Here's how the part is built. I have some questions about the finished solid (model axes, mm). Face numbers are marked on the shaded views. A direction names the side the tool comes from. Give positions to 0.01 mm unless a question says otherwise; leave off trailing zeros. Write each loop counter-clockwise with the first axis right and the second up, starting at its lowest first coordinate (ties: lowest second). Pieces come first, ordered by that corner, then holes. Notation, with made-up numbers: (-12.75, 10.25) - (-4.75, 10.25) arc R11 ccw to (-4.75, 19.25) - close; hole circle Ø8 at (54, 16). An arc over 180 degrees is marked (long way). Use a Markdown table: item, result.
```python
from build123d import *

# Parameters (mm, degrees)
SKETCH_1_R      = 1.49999994
SKETCH_1_R_2    = 9.999999603
SKETCH_1_R_3    = 2.499999901
EXTRUDE_1_DEPTH = 1.5
SKETCH_2_W      = 1.5
SKETCH_2_H      = 360
EXTRUDE_2_DEPTH = 25


with BuildPart() as part:
    # 草图1 → 凸台-拉伸1 (new body)
    with BuildSketch(Plane.XY):
        with BuildLine():
            Line((124.999995033, 180), (124.999995033, -180))
            Line((124.999995033, -180), (123.499999503, -180))
            Line((123.499999503, -180), (109.999999801, -180))
            ThreePointArc((109.999999801, -180), (106.464466036, -178.535533964), (105, -175.000000199))
            Line((105, -175.000000199), (105, -112.999998311))
            ThreePointArc((105, -112.999998311), (103.535533964, -109.464464546), (100.000000199, -107.99999851))
            Line((100.000000199, -107.99999851), (-250.16001102, -107.99999851))
            ThreePointArc((-250.16001102, -107.99999851), (-253.695544785, -109.464464546), (-255.160010821, -112.999998311))
            Line((-255.160010821, -112.999998311), (-255.160010821, -167.500000497))
            Line((-255.160010821, -167.500000497), (-255.160010821, -175.000000199))
            ThreePointArc((-255.160010821, -175.000000199), (-256.624476857, -178.535533964), (-260.160010622, -180))
            Line((-260.160010622, -180), (-273.660010324, -180))
            Line((-273.660010324, -180), (-275.160005854, -180))
            Line((-275.160005854, -180), (-275.160005854, 180))
            Line((-275.160005854, 180), (-273.660010324, 180))
            Line((-273.660010324, 180), (-260.160010622, 180))
            ThreePointArc((-260.160010622, 180), (-256.624476857, 178.535533964), (-255.160010821, 175.000000199))
            Line((-255.160010821, 175.000000199), (-255.160010821, 112.999998311))
            ThreePointArc((-255.160010821, 112.999998311), (-253.695544785, 109.464464546), (-250.16001102, 107.99999851))
            Line((-250.16001102, 107.99999851), (100.000000199, 107.99999851))
            ThreePointArc((100.000000199, 107.99999851), (103.535533964, 109.464464546), (105, 112.999998311))
            Line((105, 112.999998311), (105, 175.000000199))
            ThreePointArc((105, 175.000000199), (106.464466036, 178.535533964), (109.999999801, 180))
            Line((109.999999801, 180), (123.499999503, 180))
            Line((123.499999503, 180), (124.999995033, 180))
        make_face()
        with Locations((-201.080000404, 97.999998907)):
            Circle(SKETCH_1_R, mode=Mode.SUBTRACT)
        with Locations((-170.080001635, 97.999998907)):
            Circle(SKETCH_1_R, mode=Mode.SUBTRACT)
        Circle(SKETCH_1_R_2, mode=Mode.SUBTRACT)
        with Locations((114.99999543, 31.999998728)):
            Circle(SKETCH_1_R, mode=Mode.SUBTRACT)
        with Locations((82.999996702, 31.999998728)):
            Circle(SKETCH_1_R, mode=Mode.SUBTRACT)
        with Locations((19.919990815, 97.999998907)):
            Circle(SKETCH_1_R, mode=Mode.SUBTRACT)
        with Locations((50.919989583, 97.999998907)):
            Circle(SKETCH_1_R, mode=Mode.SUBTRACT)
        with Locations((19.919990815, 67.000000139)):
            Circle(SKETCH_1_R, mode=Mode.SUBTRACT)
        with Locations((50.919989583, 67.000000139)):
            Circle(SKETCH_1_R, mode=Mode.SUBTRACT)
        with Locations((-201.080000404, -97.999998907)):
            Circle(SKETCH_1_R, mode=Mode.SUBTRACT)
        with Locations((-170.080001635, -97.999998907)):
            Circle(SKETCH_1_R, mode=Mode.SUBTRACT)
        with Locations((19.919990815, -97.999998907)):
            Circle(SKETCH_1_R, mode=Mode.SUBTRACT)
        with Locations((50.919989583, -97.999998907)):
            Circle(SKETCH_1_R, mode=Mode.SUBTRACT)
        with Locations((114.99999543, -31.999998728)):
            Circle(SKETCH_1_R, mode=Mode.SUBTRACT)
        with Locations((82.999996702, -31.999998728)):
            Circle(SKETCH_1_R, mode=Mode.SUBTRACT)
        with Locations((-107.080004139, 97.999998907)):
            Circle(SKETCH_1_R, mode=Mode.SUBTRACT)
        with Locations((-107.080004139, 66.000000179)):
            Circle(SKETCH_1_R, mode=Mode.SUBTRACT)
        with Locations((-43.080006682, 97.999998907)):
            Circle(SKETCH_1_R, mode=Mode.SUBTRACT)
        with Locations((-43.080006682, 66.000000179)):
            Circle(SKETCH_1_R, mode=Mode.SUBTRACT)
        with Locations((-107.080004139, -97.999998907)):
            Circle(SKETCH_1_R, mode=Mode.SUBTRACT)
        with Locations((-107.080004139, -66.000000179)):
            Circle(SKETCH_1_R, mode=Mode.SUBTRACT)
        with Locations((-43.080006682, -97.999998907)):
            Circle(SKETCH_1_R, mode=Mode.SUBTRACT)
        with Locations((-43.080006682, -66.000000179)):
            Circle(SKETCH_1_R, mode=Mode.SUBTRACT)
        with Locations((-201.080000404, 67.000000139)):
            Circle(SKETCH_1_R, mode=Mode.SUBTRACT)
        with Locations((-170.080001635, 67.000000139)):
            Circle(SKETCH_1_R, mode=Mode.SUBTRACT)
        with Locations((-201.080000404, -67.000000139)):
            Circle(SKETCH_1_R, mode=Mode.SUBTRACT)
        with Locations((-170.080001635, -67.000000139)):
            Circle(SKETCH_1_R, mode=Mode.SUBTRACT)
        with Locations((19.919990815, -67.000000139)):
            Circle(SKETCH_1_R, mode=Mode.SUBTRACT)
        with Locations((50.919989583, -67.000000139)):
            Circle(SKETCH_1_R, mode=Mode.SUBTRACT)
        with Locations((-196.080000602, 97.999998907)):
            Circle(SKETCH_1_R, mode=Mode.SUBTRACT)
        with Locations((-196.080000602, 84.999999424)):
            Circle(SKETCH_1_R, mode=Mode.SUBTRACT)
        with Locations((-170.080001635, 84.999999424)):
            Circle(SKETCH_1_R, mode=Mode.SUBTRACT)
        with Locations((45.919989781, 97.999998907)):
            Circle(SKETCH_1_R, mode=Mode.SUBTRACT)
        with Locations((19.919990815, 84.999999424)):
            Circle(SKETCH_1_R, mode=Mode.SUBTRACT)
        with Locations((45.919989781, 84.999999424)):
            Circle(SKETCH_1_R, mode=Mode.SUBTRACT)
        with Locations((-196.080000602, -97.999998907)):
            Circle(SKETCH_1_R, mode=Mode.SUBTRACT)
        with Locations((-196.080000602, -84.999999424)):
            Circle(SKETCH_1_R, mode=Mode.SUBTRACT)
        with Locations((-170.080001635, -84.999999424)):
            Circle(SKETCH_1_R, mode=Mode.SUBTRACT)
        with Locations((45.919989781, -97.999998907)):
            Circle(SKETCH_1_R, mode=Mode.SUBTRACT)
        with Locations((19.919990815, -84.999999424)):
            Circle(SKETCH_1_R, mode=Mode.SUBTRACT)
        with Locations((45.919989781, -84.999999424)):
            Circle(SKETCH_1_R, mode=Mode.SUBTRACT)
        with Locations((-19.999999205, 9.999999603)):
            Circle(SKETCH_1_R_3, mode=Mode.SUBTRACT)
        with Locations((-19.999999205, -9.999999603)):
            Circle(SKETCH_1_R_3, mode=Mode.SUBTRACT)
        with Locations((19.999999205, 9.999999603)):
            Circle(SKETCH_1_R_3, mode=Mode.SUBTRACT)
        with Locations((19.999999205, -9.999999603)):
            Circle(SKETCH_1_R_3, mode=Mode.SUBTRACT)
        with Locations((-265.160006251, 31.999998728)):
            Circle(SKETCH_1_R, mode=Mode.SUBTRACT)
        with Locations((-233.160007523, 31.999998728)):
            Circle(SKETCH_1_R, mode=Mode.SUBTRACT)
        with Locations((-201.160008794, 31.999998728)):
            Circle(SKETCH_1_R, mode=Mode.SUBTRACT)
        with Locations((-201.160008794, 0)):
            Circle(SKETCH_1_R, mode=Mode.SUBTRACT)
        with Locations((-265.160006251, -31.999998728)):
            Circle(SKETCH_1_R, mode=Mode.SUBTRACT)
        with Locations((-233.160007523, -31.999998728)):
            Circle(SKETCH_1_R, mode=Mode.SUBTRACT)
        with Locations((-201.160008794, -31.999998728)):
            Circle(SKETCH_1_R, mode=Mode.SUBTRACT)
        with Locations((-130.160011616, 9.999999603)):
            Circle(SKETCH_1_R_3, mode=Mode.SUBTRACT)
        with Locations((-130.160011616, -9.999999603)):
            Circle(SKETCH_1_R_3, mode=Mode.SUBTRACT)
        with Locations((-169.160010066, 31.999998728)):
            Circle(SKETCH_1_R, mode=Mode.SUBTRACT)
        with Locations((-169.160010066, 0)):
            Circle(SKETCH_1_R, mode=Mode.SUBTRACT)
        with Locations((-169.160010066, -31.999998728)):
            Circle(SKETCH_1_R, mode=Mode.SUBTRACT)
        with Locations((-265.160006251, 0)):
            Circle(SKETCH_1_R, mode=Mode.SUBTRACT)
        with Locations((-233.160007523, 0)):
            Circle(SKETCH_1_R, mode=Mode.SUBTRACT)
        with Locations((50.999997973, 31.999998728)):
            Circle(SKETCH_1_R, mode=Mode.SUBTRACT)
        with Locations((50.999997973, 0)):
            Circle(SKETCH_1_R, mode=Mode.SUBTRACT)
        with Locations((50.999997973, -31.999998728)):
            Circle(SKETCH_1_R, mode=Mode.SUBTRACT)
        with Locations((-110.83000399, 34.00000145)):
            Circle(SKETCH_1_R, mode=Mode.SUBTRACT)
        with Locations((-78.830005261, 34.00000145)):
            Circle(SKETCH_1_R, mode=Mode.SUBTRACT)
        with Locations((-46.830006533, 34.00000145)):
            Circle(SKETCH_1_R, mode=Mode.SUBTRACT)
        with Locations((-110.83000399, -34.00000145)):
            Circle(SKETCH_1_R, mode=Mode.SUBTRACT)
        with Locations((-78.830005261, -34.00000145)):
            Circle(SKETCH_1_R, mode=Mode.SUBTRACT)
        with Locations((-46.830006533, -34.00000145)):
            Circle(SKETCH_1_R, mode=Mode.SUBTRACT)
    extrude(amount=EXTRUDE_1_DEPTH)

    # 草图2 → 凸台-拉伸2 (add)
    with BuildSketch(Plane.XY.offset(1.5)):
        with Locations((124.249995033, 0)):
            Rectangle(SKETCH_2_W, SKETCH_2_H)
        with Locations((-274.410005854, 0)):
            Rectangle(SKETCH_2_W, SKETCH_2_H)
    extrude(amount=-EXTRUDE_2_DEPTH)


solid = part.part
```
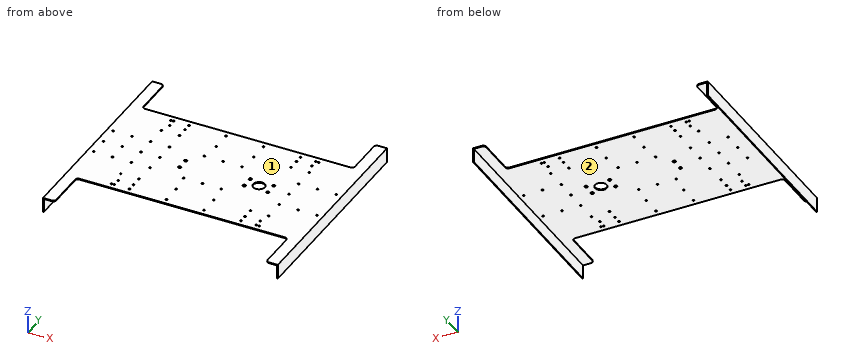
Item 1: I need wall thicknesses on line 1 along X through (y, z) = (-65, -10.25); line 2 along Z through (x, y) = (-28, -86.5). Which ranges of each line are inside material? Lowest first, please. Write a range as [from, to].
Values:
| item | result |
|---|---|
| line 1 | x = [-275.16, -273.66], [123.5, 125] |
| line 2 | z = [0, 1.5] |
Item 2: Will these pins go through, and if not, where does the flat tip stop? pin 1 Ø2 at (x, y) = (-218, 59.5) entering from -Z; pin 2 Ø4 at (x, y) = (-114.5, 110.5) entering from +Z (3 decimals); pin 3 Ø2 at (x, y) = (50, -67.5) entering from +Z; pin 4 Ø1.6 at (x, z) = (-130, 0.5) entering from -Y.
Values:
| item | result |
|---|---|
| pin 1 | stops at z = 0 |
| pin 2 | passes through |
| pin 3 | stops at z = 1.5 |
| pin 4 | stops at y = -108 |
Item 3: If we section it at B-B, the plane z = -8: Write out the boundary of the cut face in (x, y).
Values:
| item | result |
|---|---|
| outline | (-275.16, -180) - (-273.66, -180) - (-273.66, 180) - (-275.16, 180) - close; (123.5, -180) - (125, -180) - (125, 180) - (123.5, 180) - close |
Item 4: If we section it at C-C, the plane x = -152.5: Write out the boundary of the cut face in (y, z).
Values:
| item | result |
|---|---|
| outline | (-108, 0) - (108, 0) - (108, 1.5) - (-108, 1.5) - close |
Item 5: For the marked faces 1 and 2, which set-ups out of +Z, -Z, +X, -X, +Y, -Y let a thin tool reach every point of the face, with its end or its side?
Values:
| item | result |
|---|---|
| face 1 | +Z, +X, -X, +Y, -Y |
| face 2 | -Z, +Y, -Y |
Item 6: If we section it at A-A, the plane y = -119.5: Write out the boundary of the cut face in (x, z), plus the area to 4 significant figures.
Values:
| item | result |
|---|---|
| outline | (-275.16, -23.5) - (-273.66, -23.5) - (-273.66, 0) - (-255.16, 0) - (-255.16, 1.5) - (-275.16, 1.5) - close; (105, 0) - (123.5, 0) - (123.5, -23.5) - (125, -23.5) - (125, 1.5) - (105, 1.5) - close |
| area | 130.5 mm2 |
